Geometry: final body of the model. Coordinates: model frame, mm. A direction names the side the tool comes from. Coordinates: 2 decimals unless noted, no trailing zeros. Loops run counter-clockwise (first coordinate to the right, second up) from the corner with the lowest first, then second, coordinate; pieces in that order, holes last. Notation, with made-up numbers: (58.25, 76.5) - (95.25, 76.5) arc R24 ccw to (95.25, 105.5) - close; hole circle Ø7 at (60, -8.5). An arc over 180 degrees is marked (long way). Put each result on its own line as item: value. Start each with the question number.
1) Section D-D on z = 5. Output: boundary loops of the cut face in (x, y) (3 decimals).
2) Reachability of faces 4 (the flat face through (-5, 11, 6.985)), 5 (the flat face through (-1, 20.955, 6)), 6 (the flat face through (7.62, 7, 6)) from +Z, -Z, +X, -X, +Y, -Y: full face, straight path, thin tool, end or side. Return the list, or none.
3) Section A-A on x = 18. Output: boundary loops of the cut face in (y, z).
4) Contact query for flat-ended pins moving along their axis: pin 1 Ø6.5 at (x, z) = (12, 7.5) entering from -Y; pin 2 Ø5 at (y, z) = (17, 1.5) entering from -X (3 decimals); pin 3 Ø6 at (x, z) = (21.5, 7.5) entering from -Y. Output: stop coordinate, or through.
5) Section B-B on y = 14.75. Output: boundary loops of the cut face in (x, z) (3 decimals).
6) Material intervals for line 1 along Y through (x, z) = (19, 1.75); line 2 along X through (y, z) = (7.5, 0.75); line 3 along X through (y, z) = (20, 7.25) (3 decimals), sorted ascending. Write a range as from..to.
7) Section C-C on z = 11.25. Output: boundary loops of the cut face in (x, y) (3 decimals).
8) Draft query along X for faces 1 (the cylindrical face through (6.7, -1.6, 6.4)), 2 (the flat face through (-7.62, 11, 6)), 3 (the cylindrical face through (5.99, 18.1, 6.44)). Return one class per face: +X half, -X half, draft (parallel to the pull), parting line (faces both ways), or undercut.
```python
from build123d import *

# Parameters (mm, degrees)
F1_DEPTH = 12.7
F2_R     = 3.175
F3_W     = 20.32
F3_H     = 1.27
F4_DEPTH = 7.62
F5_SIZE  = 2.54


with BuildPart() as f1:
    # F0 (on Top) → F1 (new body)
    with BuildSketch(Plane.XY):
        Polygon((0, 24.13), (0, -2.194877), (0, -2.54), (7.62, -2.54), (7.62, 16.51), (26.67, 16.51), (26.67, 24.13), align=None)
        Polygon((5.08, 0), (2.54, 0), (2.54, 21.59), (5.08, 21.59), (24.13, 21.59), (24.13, 19.05), (5.08, 19.05), align=None, mode=Mode.SUBTRACT)
    extrude(amount=F1_DEPTH)

    # F2
    f2_edges = [f1.edges().sort_by_distance(p)[0] for p in [
        (26.67, 24.13, 6.35),
        (26.67, 16.51, 6.35),
        (5.08, 19.05, 6.35),
        (0, 24.13, 6.35),
        (7.62, -2.54, 6.35),
        (0, -2.54, 6.35),
        (7.62, 16.51, 6.35),
    ]]
    fillet(f2_edges, radius=F2_R)

    # F3 (on face) → F4 (join)
    with BuildSketch(Plane(origin=(0, 0, 0), x_dir=(0, -1, 0), z_dir=(-1, 0, 0))):
        with Locations((-10.795, 6.35)):
            Rectangle(F3_W, F3_H)
    extrude(amount=F4_DEPTH)

    # F5
    f5_edges = [f1.edges().sort_by_distance(p)[0] for p in [
        (0, 10.795, 5.715),
        (0, 10.795, 6.985),
        (-7.62, 20.955, 6.35),
        (-7.62, 0.635, 6.35),
    ]]
    chamfer(f5_edges, length=F5_SIZE)


solid = f1.part
```
Answer block:
1. outline: (-1.825, 0.635) - (0, 0.635) arc R3.175 ccw to (3.175, -2.54) - (4.445, -2.54) arc R3.175 ccw to (7.62, 0.635) - (7.62, 13.335) arc R3.175 cw to (10.795, 16.51) - (23.495, 16.51) arc R3.175 ccw to (26.67, 19.685) - (26.67, 20.955) arc R3.175 ccw to (23.495, 24.13) - (3.175, 24.13) arc R3.175 ccw to (0, 20.955) - (-1.825, 20.955) - close; hole (2.54, 0) - (5.08, 0) - (5.08, 15.875) arc R3.175 cw to (8.255, 19.05) - (24.13, 19.05) - (24.13, 21.59) - (2.54, 21.59) - close
2. face 4: +Z, -X, +Y, -Y
2. face 5: +Z, -Z, -X, +Y
2. face 6: +Z, -Z, +X, -Y
3. outline: (16.51, 0) - (19.05, 0) - (19.05, 12.7) - (16.51, 12.7) - close; (21.59, 0) - (24.13, 0) - (24.13, 12.7) - (21.59, 12.7) - close
4. pin 1: stops at y = 15.76
4. pin 2: stops at x = -0.825
4. pin 3: stops at y = 16.51
5. outline: (-7.62, 5.715) - (-2.54, 5.715) - (0, 3.175) - (0, 0) - (2.54, 0) - (2.54, 12.7) - (0, 12.7) - (0, 9.525) - (-2.54, 6.985) - (-7.62, 6.985) - close; (5.08, 0) - (7.953, 0) - (7.953, 12.7) - (5.08, 12.7) - close
6. line 1: y = 16.51..19.05, 21.59..24.13
6. line 2: x = 0..2.54, 5.08..7.62
6. line 3: x = -2.275..2.54, 24.13..26.67
7. outline: (0, 0.635) arc R3.175 ccw to (3.175, -2.54) - (4.445, -2.54) arc R3.175 ccw to (7.62, 0.635) - (7.62, 13.335) arc R3.175 cw to (10.795, 16.51) - (23.495, 16.51) arc R3.175 ccw to (26.67, 19.685) - (26.67, 20.955) arc R3.175 ccw to (23.495, 24.13) - (3.175, 24.13) arc R3.175 ccw to (0, 20.955) - close; hole (2.54, 0) - (5.08, 0) - (5.08, 15.875) arc R3.175 cw to (8.255, 19.05) - (24.13, 19.05) - (24.13, 21.59) - (2.54, 21.59) - close
8. face 1: +X half
8. face 2: -X half
8. face 3: undercut
